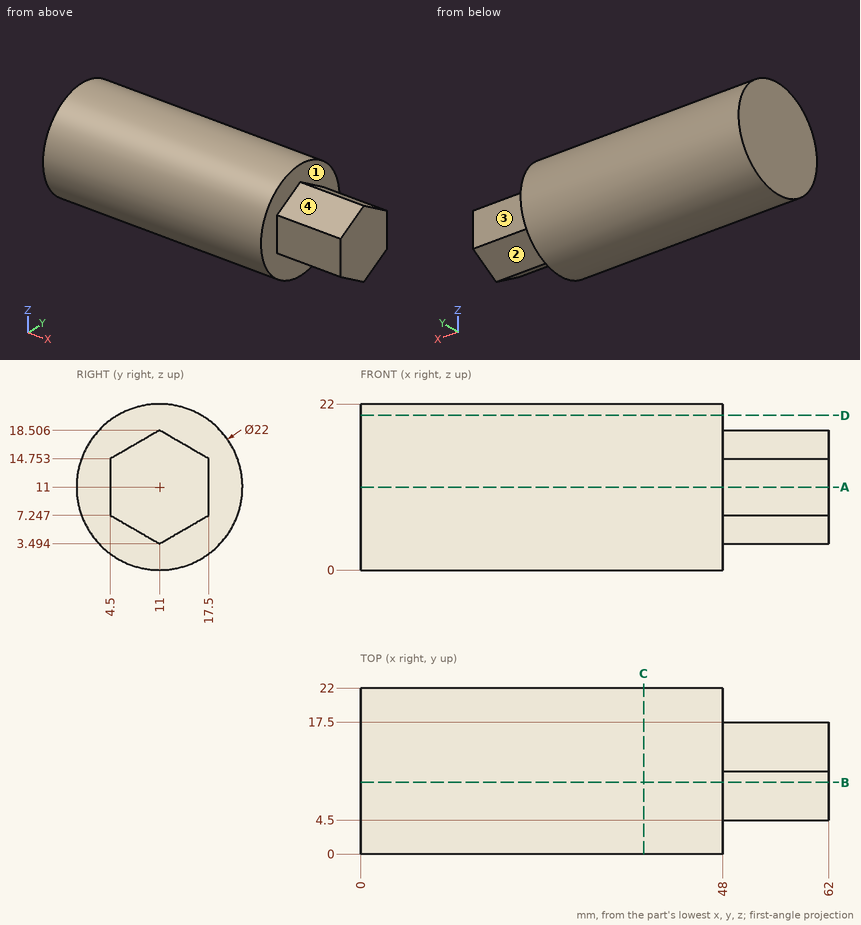
Verification items for this drawing (mm, ordinates from the low corner). A direction names the side the tool comes from. Coordinates: 2 decimals unless noted, no trailing zeros. Order: outer loops, then holes, each group sorted by start corner. A loop starts at its lowest first (then second) coordinate and runs counter-clockwise, first axis right, second up. Notation, with made-up numbers: (-19, -13) - (11, -13) arc R9 ccw to (11, 2) - close; hole circle Ø9 at (31, 73). An arc over 180 degrees is marked (long way). Use one line per item in the form item = value.
1. Section check C-C (x = 37.5). Record the boundary of the cut face in (y, z).
Here are the results:
outline = circle Ø22 at (11, 11)
2. Section check D-D (z = 20.5). Record the boundary of the cut face in (x, y) (1 decimal).
Here are the results:
outline = (0, 5.5) - (48, 5.5) - (48, 16.5) - (0, 16.5) - close
3. Gauge pin test, flat ends, axial feed: pin 1 (8.5 mm diameter, centred on x = 54.5, z = 11, fed in from -Y); pin 2 (6 mm diameter, centred on x = 12.5, z = 18, fed in from +Y); pin 3 (2 mm diameter, centred on x = 42, z = 6, fed in from -Y). Record the tip position at first contact, or that the pin passes through.
Here are the results:
pin_1 = 4.5
pin_2 = 21.25
pin_3 = 0.75
4. Scan lines: line 1 (X direction, y = 7.5, z = 2.5); line 2 (Y direction, x = 10.5, z = 11); line 3 (Z direction, x = 49, y = 16.5). Record each from-to range of solid material in increasing order.
Here are the results:
line_1 = 0 to 48
line_2 = 0 to 22
line_3 = 6.67 to 15.33
5. Access from +Z, -Z, +X, -X, +Y, -Y to the whole of each face (thin tool, end or side, straight path). Record for the marked faces 1, 2, 3 and 4.
Here are the results:
face_1 = +X
face_2 = -Z, +X, +Y
face_3 = +Z, -Z, +X, +Y
face_4 = +Z, +X, -Y
6. Section check B-B (y = 9.5). Record the boundary of the cut face in (x, z), then the cut area to 3 significant figures.
Here are the results:
outline = (0, 0.1) - (48, 0.1) - (48, 4.36) - (62, 4.36) - (62, 17.64) - (48, 17.64) - (48, 21.9) - (0, 21.9) - close
area = 1,230 mm²
7. Section check A-A (z = 11). Record the boundary of the cut face in (x, y).
Here are the results:
outline = (0, 0) - (48, 0) - (48, 4.5) - (62, 4.5) - (62, 17.5) - (48, 17.5) - (48, 22) - (0, 22) - close
